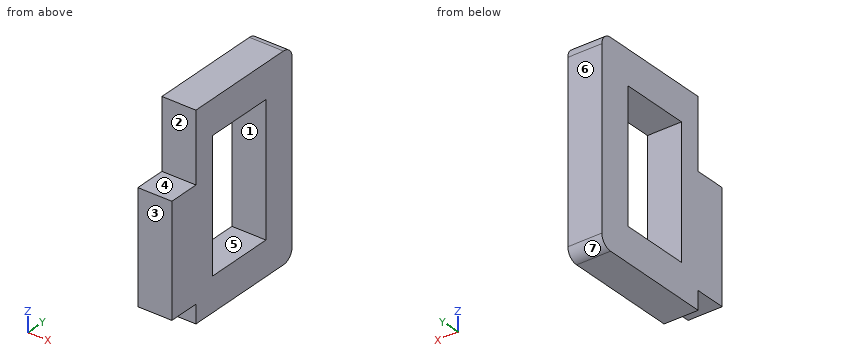
from build123d import *

# Parameters (mm, degrees)
SKETCH1_W           = 23
SKETCH1_H           = 12.2
BOSS_EXTRUDE1_DEPTH = 6
FILLET1_R           = 2


with BuildPart() as part:
    # Sketch1 → Boss-Extrude1 (new body)
    with BuildSketch(Plane(origin=(0, 0, 0), x_dir=(0, 0, -1), z_dir=(1, 0, 0))):
        Polygon((17.5, -9.9), (17.5, 12.1), (-17.5, 12.1), (-17.5, -9.9), (-5.25, -9.9), (-5.25, -15.4), (14.25, -15.4), (14.25, -9.9), align=None)
        Rectangle(SKETCH1_W, SKETCH1_H, mode=Mode.SUBTRACT)
    extrude(amount=BOSS_EXTRUDE1_DEPTH)

    # Fillet1
    fillet1_edges = [part.edges().sort_by_distance(p)[0] for p in [
        (3, 12.1, -17.5),
        (3, 12.1, 17.5),
    ]]
    fillet(fillet1_edges, radius=FILLET1_R)


solid = part.part
The model under review builds one solid part; all positions refer to its coordinate system, in mm. Face numbers are marked on the shaded views. A direction names the side the tool comes from. Coordinates: 2 decimals unless noted, no trailing zeros. Write each loop counter-clockwise with the first axis right and the second up, starting at its lowest first coordinate (ties: lowest second). Pieces come first, ordered by that corner, then holes. Notation, with made-up numbers: M -1.5,6.5 L 51.5,6.5 A21 ccw 51.5,33.5 Z; hole C -25,73.5 d4. An arc over 180 degrees is marked long. Put each result on its own line as item: value.
1) Add section B-B on x = 5.25. Give the boundary of the cut face in (y, z), then the cut area to 3 significant figures.
Computed:
outline: M -15.4,-14.25 L -9.9,-14.25 L -9.9,-17.5 L 10.1,-17.5 A2 ccw 12.1,-15.5 L 12.1,15.5 A2 ccw 10.1,17.5 L -9.9,17.5 L -9.9,5.25 L -15.4,5.25 Z; hole M -6.1,-11.5 L 6.1,-11.5 L 6.1,11.5 L -6.1,11.5 Z
area: 595 mm2
2) Add section C-C on y = 1.25. Give the boundary of the cut face in (x, z).
Computed:
outline: M 0,-17.5 L 6,-17.5 L 6,-11.5 L 0,-11.5 Z; M 0,11.5 L 6,11.5 L 6,17.5 L 0,17.5 Z
3) Add section D-D on y = -11. Give the boundary of the cut face in (x, z).
Computed:
outline: M 0,-14.25 L 6,-14.25 L 6,5.25 L 0,5.25 Z
4) Add section A-A on z = 8.5. Give the boundary of the cut face in (x, y), then the cut area to 3 significant figures.
Computed:
outline: M 0,-9.9 L 6,-9.9 L 6,-6.1 L 0,-6.1 Z; M 0,6.1 L 6,6.1 L 6,12.1 L 0,12.1 Z
area: 58.8 mm2
5) For the marked faces 1, 2 and 3, list the 3-axis set-ups (+Z, -Z, +X, -X, +Y, -Y) from which the entire face can be reached by the end or side of a thin tool; tool diameter is ignored.
Computed:
face 1: +X, -X
face 2: +Z, +X, -X, -Y
face 3: +Z, -Z, +X, -X, -Y
6) Draft analysis for pull direction Z (two halves, no side actions). For the marked faces 4, 5, 6 and 7, state which applies: released by +Z, released by -Z, zero draft, split by the parting line, or undercut.
Computed:
face 4: released by +Z
face 5: undercut
face 6: zero draft
face 7: released by -Z
7) Wall thickness on probe 1 along Z at (x, y) = (3.3, 3); probe 2 along Y at (x, z) = (2.6, -10); probe 3 along Y at (x, z) = (5.2, 14.5): over which ranges is each line inside the solid? List them lowest first. Write a range as [from, to].
Computed:
probe 1: z = [-17.5, -11.5], [11.5, 17.5]
probe 2: y = [-15.4, -6.1], [6.1, 12.1]
probe 3: y = [-9.9, 12.1]
